from build123d import *

# Parameters (mm, degrees)
SKETCH1_R           = 17
BOSS_EXTRUDE1_DEPTH = 14
CUT_EXTRUDE2_REACH  = 29.821
SKETCH3_R           = 2.5
BOSS_EXTRUDE2_START = 10
SKETCH5_R           = 8.5
SKETCH5_R_2         = 2.5
BOSS_EXTRUDE2_DEPTH = 10
BOSS_EXTRUDE3_DEPTH = 24
SKETCH7_R           = 17
SKETCH7_R_2         = 14
CUT_EXTRUDE5_DEPTH  = 5
SKETCH8_R           = 2
CUT_EXTRUDE6_DEPTH  = 5


with BuildPart() as part:
    # Sketch1 → Boss-Extrude1 (new body)
    with BuildSketch(Plane.XY):
        Circle(SKETCH1_R)
    extrude(amount=BOSS_EXTRUDE1_DEPTH)

    # Sketch3 → Cut-Extrude2 (cut, up to next)
    with BuildSketch(Plane.XY.offset(14), mode=Mode.PRIVATE) as cut_extrude2_sk1:
        Circle(SKETCH3_R)
    cut_extrude2_tool1 = extrude(cut_extrude2_sk1.sketch, amount=-CUT_EXTRUDE2_REACH, mode=Mode.PRIVATE) & part.part
    add(cut_extrude2_tool1.solids().sort_by_distance((0, 0, 14))[0], mode=Mode.SUBTRACT)

    # Sketch5 → Boss-Extrude2 (add)
    with BuildSketch(Plane.XY.offset(14).offset(BOSS_EXTRUDE2_START)):
        Circle(SKETCH5_R)
        Circle(SKETCH5_R_2, mode=Mode.SUBTRACT)
    extrude(amount=-BOSS_EXTRUDE2_DEPTH)

    # Sketch6 → Boss-Extrude3 (add)
    with BuildSketch(Plane.XY.offset(24)):
        with BuildLine():
            Line((1.5, 2), (-1.5, 2))
            ThreePointArc((-1.5, 2), (0, 2.5), (1.5, 2))
        make_face()
    extrude(amount=-BOSS_EXTRUDE3_DEPTH)

    # Sketch7 → Cut-Extrude5 (cut, symmetric)
    with BuildSketch(Plane(origin=(0, 0, 7), x_dir=(-1, 0, 0), z_dir=(0, 0, -1))):
        Circle(SKETCH7_R)
        Circle(SKETCH7_R_2, mode=Mode.SUBTRACT)
    extrude(amount=CUT_EXTRUDE5_DEPTH, both=True, mode=Mode.SUBTRACT)

    # Sketch8 → Cut-Extrude6 (cut, symmetric)
    with BuildSketch(Plane(origin=(0, 0, 7), x_dir=(-1, 0, 0), z_dir=(0, 0, -1))):
        with Locations((0, 14)):
            Circle(SKETCH8_R)
        with Locations((4.788282007, 13.155696691)):
            Circle(SKETCH8_R)
        with Locations((8.999026536, 10.724622204)):
            Circle(SKETCH8_R)
        with Locations((12.124355653, 7)):
            Circle(SKETCH8_R)
        with Locations((13.787308542, 2.431074487)):
            Circle(SKETCH8_R)
        with Locations((13.787308542, -2.431074487)):
            Circle(SKETCH8_R)
        with Locations((12.124355653, -7)):
            Circle(SKETCH8_R)
        with Locations((8.999026536, -10.724622204)):
            Circle(SKETCH8_R)
        with Locations((4.788282007, -13.155696691)):
            Circle(SKETCH8_R)
        with Locations((0, -14)):
            Circle(SKETCH8_R)
        with Locations((-4.788282007, -13.155696691)):
            Circle(SKETCH8_R)
        with Locations((-8.999026536, -10.724622204)):
            Circle(SKETCH8_R)
        with Locations((-12.124355653, -7)):
            Circle(SKETCH8_R)
        with Locations((-13.787308542, -2.431074487)):
            Circle(SKETCH8_R)
        with Locations((-13.787308542, 2.431074487)):
            Circle(SKETCH8_R)
        with Locations((-12.124355653, 7)):
            Circle(SKETCH8_R)
        with Locations((-8.999026536, 10.724622204)):
            Circle(SKETCH8_R)
        with Locations((-4.788282007, 13.155696691)):
            Circle(SKETCH8_R)
    extrude(amount=CUT_EXTRUDE6_DEPTH, both=True, mode=Mode.SUBTRACT)


solid = part.part
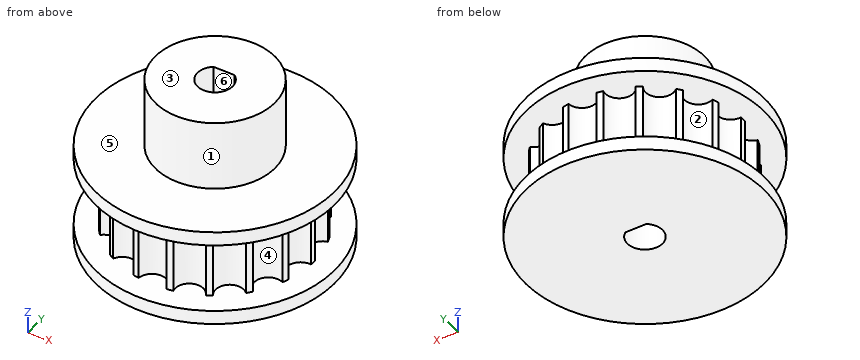
Verification items for the finished model (mm, model axes). Face numbers are marked on the shaded views. A direction names the side the tool comes from. Give positions to 0.01 mm unless a question says otherwise; leave off trailing zeros. Write each loop counter-clockwise with the first axis right and the second up, starting at its lowest first coordinate (ties: lowest second). Pieces come first, ordered by that corner, then holes. Notation, with made-up numbers: M 18,37 L 23,37 A11 ccw 23,45 Z; hole C 70,2 d8. An arc over 180 degrees is marked long. Write item = value, one per line.
(1) Sectioned sample at B-B (x = 0). Record the cut outline in (y, z).
Found:
outline = M -17,0 L -2.5,0 L -2.5,24 L -8.5,24 L -8.5,14 L -17,14 L -17,12 L -12,12 L -12,2 L -17,2 Z; M 2,0 L 17,0 L 17,2 L 12,2 L 12,12 L 17,12 L 17,14 L 8.5,14 L 8.5,24 L 2,24 Z
(2) Sectioned sample at D-D (x = -4.5). Record the cut outline in (y, z), then the cut area to 3 significant figures.
Found:
outline = M -16.39,0 L 16.39,0 L 16.39,2 L 11.18,2 L 11.18,12 L 16.39,12 L 16.39,14 L 7.21,14 L 7.21,24 L -7.21,24 L -7.21,14 L -16.39,14 L -16.39,12 L -11.18,12 L -11.18,2 L -16.39,2 Z
area = 499 mm2
(3) Draft check along X on the marked faces 1, 2 and 3. Enter one of: released by +X, released by -X, zero draft, split by the parting line, or undercut.
Found:
face_1 = split by the parting line
face_2 = undercut
face_3 = zero draft
(4) Sectioned sample at A-A (y = 0). Record the cut outline in (x, z), then the cut area to 3 significant figures.
Found:
outline = M -17,0 L -2.5,0 L -2.5,24 L -8.5,24 L -8.5,14 L -17,14 L -17,12 L -14,12 L -14,2 L -17,2 Z; M 2.5,0 L 17,0 L 17,2 L 14,2 L 14,12 L 17,12 L 17,14 L 8.5,14 L 8.5,24 L 2.5,24 Z
area = 466 mm2
(5) Material ranges on line 1 (X direction, y = 0, z = 9.25); line 2 (Z direction, x = -7.5, y = 11); line 3 (Z direction, x = 11, y = -4), recorded low to high.
Found:
line_1 = -14 to -2.5, 2.5 to 14
line_2 = 0 to 2, 12 to 14
line_3 = 0 to 14
(6) Access from +Z, -Z, +X, -X, +Y, -Y to the whole of each face (thin tool, end or side, straight path). Record for the marked faces 4, 5 and 6.
Found:
face_4 = none
face_5 = +Z
face_6 = +Z, -Z
(7) Go/stop test with flat-tipped pins: pin 1 Ø3.5 at (x, z) = (0, 8) entering from -Y; pin 2 Ø6 at (x, y) = (0, 0) entering from +Z; pin 3 Ø1.5 at (x, z) = (-6, 18) entering from +Y; pin 4 Ø2 at (y, z) = (-6.5, 17) entering from -X. Record where each tip stops, or that it passes through.
Found:
pin_1 = -13.03
pin_2 = 24
pin_3 = 6.68
pin_4 = -6.48
(8) Sectioned sample at C-C (x = 9.5). Record the cut outline in (y, z).
Found:
outline = M -14.1,0 L 14.1,0 L 14.1,2 L 8.79,2 L 8.79,12 L 14.1,12 L 14.1,14 L -14.1,14 L -14.1,12 L -8.79,12 L -8.79,2 L -14.1,2 Z
